The model under review builds one solid part; all positions refer to its coordinate system, in mm. Face numbers are marked on the shaded views. Give positions to 0.01 mm unless a question says otherwise; leave off trailing zeros. Loops run counter-clockwise (first coordinate to the right, second up) from the corner with the lowest first, then second, coordinate; pieces in that order, holes last. Notation, with made-up numbers: (28, 68.25) - (69, 68.25) arc R22 cw to (69, 106.25) - close; hole circle Ø2 at (-22.5, 87.5). An arc over 180 degrees is marked (long way). Return JSON: item names as keys, results as strings. Group by question number.
from build123d import *

# Parameters (mm, degrees)
SKETCH1_W           = 98
SKETCH1_H           = 60
BOSS_EXTRUDE1_DEPTH = 1.5
SKETCH2_W           = 97
SKETCH2_H           = 39.5
BOSS_EXTRUDE2_DEPTH = 9
CUT_EXTRUDE1_DEPTH  = 1.5
CUT_EXTRUDE2_REACH  = 60.155
SKETCH4_R           = 1.5
SKETCH5_W           = 37.809406893
SKETCH5_H           = 4.525576916
BOSS_EXTRUDE3_DEPTH = 0.01


with BuildPart() as part:
    # Sketch1 → Boss-Extrude1 (new body)
    with BuildSketch(Plane(origin=(0, 0, 0), x_dir=(1, 0, 0), z_dir=(0, 1, 0))):
        Rectangle(SKETCH1_W, SKETCH1_H)
    extrude(amount=BOSS_EXTRUDE1_DEPTH)

    # Sketch2 → Boss-Extrude2 (add)
    with BuildSketch(Plane(origin=(0, 1.5, 0), x_dir=(1, 0, 0), z_dir=(0, 1, 0))):
        with Locations((0, 0.25)):
            Rectangle(SKETCH2_W, SKETCH2_H)
    extrude(amount=BOSS_EXTRUDE2_DEPTH)

    # Sketch3 → Cut-Extrude1 (cut)
    with BuildSketch(Plane(origin=(0, 10.5, 0), x_dir=(1, 0, 0), z_dir=(0, 1, 0))):
        with BuildLine():
            Line((-36, 13.25), (36, 13.25))
            ThreePointArc((36, 13.25), (37.414213562, 12.664213562), (38, 11.25))
            Line((38, 11.25), (38, -10.75))
            ThreePointArc((38, -10.75), (37.414213562, -12.164213562), (36, -12.75))
            Line((36, -12.75), (-36, -12.75))
            ThreePointArc((-36, -12.75), (-37.414213562, -12.164213562), (-38, -10.75))
            Line((-38, -10.75), (-38, 11.25))
            ThreePointArc((-38, 11.25), (-37.414213562, 12.664213562), (-36, 13.25))
        make_face()
    extrude(amount=-CUT_EXTRUDE1_DEPTH, mode=Mode.SUBTRACT)

    # Sketch4 → Cut-Extrude2 (cut, up to next)
    with BuildSketch(Plane(origin=(0, 1.5, 0), x_dir=(1, 0, 0), z_dir=(0, 1, 0)), mode=Mode.PRIVATE) as cut_extrude2_sk1:
        with Locations(Location((-46.5, 27.5, 0), (0, 0, 270))):
            Circle(SKETCH4_R)
    cut_extrude2_tool1 = extrude(cut_extrude2_sk1.sketch, amount=-CUT_EXTRUDE2_REACH, mode=Mode.PRIVATE) & part.part
    # Sketch4 → Cut-Extrude2 (cut, up to next)
    with BuildSketch(Plane(origin=(0, 1.5, 0), x_dir=(1, 0, 0), z_dir=(0, 1, 0)), mode=Mode.PRIVATE) as cut_extrude2_sk2:
        with Locations(Location((46.5, 27.5, 0), (0, 0, 270))):
            Circle(SKETCH4_R)
    cut_extrude2_tool2 = extrude(cut_extrude2_sk2.sketch, amount=-CUT_EXTRUDE2_REACH, mode=Mode.PRIVATE) & part.part
    # Sketch4 → Cut-Extrude2 (cut, up to next)
    with BuildSketch(Plane(origin=(0, 1.5, 0), x_dir=(1, 0, 0), z_dir=(0, 1, 0)), mode=Mode.PRIVATE) as cut_extrude2_sk3:
        with Locations(Location((46.5, -27.5, 0), (0, 0, 270))):
            Circle(SKETCH4_R)
    cut_extrude2_tool3 = extrude(cut_extrude2_sk3.sketch, amount=-CUT_EXTRUDE2_REACH, mode=Mode.PRIVATE) & part.part
    # Sketch4 → Cut-Extrude2 (cut, up to next)
    with BuildSketch(Plane(origin=(0, 1.5, 0), x_dir=(1, 0, 0), z_dir=(0, 1, 0)), mode=Mode.PRIVATE) as cut_extrude2_sk4:
        with Locations(Location((-46.5, -27.5, 0), (0, 0, 270))):
            Circle(SKETCH4_R)
    cut_extrude2_tool4 = extrude(cut_extrude2_sk4.sketch, amount=-CUT_EXTRUDE2_REACH, mode=Mode.PRIVATE) & part.part
    add(cut_extrude2_tool1.solids().sort_by_distance((-46.5, 1.5, -27.5))[0], mode=Mode.SUBTRACT)
    add(cut_extrude2_tool2.solids().sort_by_distance((46.5, 1.5, -27.5))[0], mode=Mode.SUBTRACT)
    add(cut_extrude2_tool3.solids().sort_by_distance((46.5, 1.5, 27.5))[0], mode=Mode.SUBTRACT)
    add(cut_extrude2_tool4.solids().sort_by_distance((-46.5, 1.5, 27.5))[0], mode=Mode.SUBTRACT)

    # Sketch5 → Boss-Extrude3 (add)
    with BuildSketch(Plane(origin=(0, 1.5, 0), x_dir=(1, 0, 0), z_dir=(0, 1, 0))):
        with Locations((-21.049918021, 27.737211542)):
            Rectangle(SKETCH5_W, SKETCH5_H)
    extrude(amount=BOSS_EXTRUDE3_DEPTH)


solid = part.part
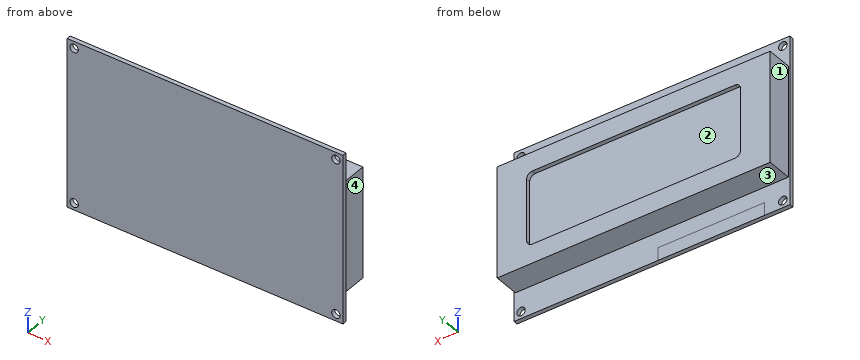
Item 1: Take a section at B-B (z = 27.5). State the section outline as (x, y) points.
Item 2: Take a section at C-C (x = 13). State the section outline as (y, z) points, then the cut area to 4 significant figures.
Item 3: Take a section at A-A (x = 46.5). State the section outline as (y, z) points, then the cut area to 4 significant figures.
Item 4: For P1, Ø3.5, axis at x = 46.5, z = 27.5, coming from the +Y side; P2, Ø4.5, axis at y = 7.5, z = 6.5, coming from the +X side; P3, Ø1, axis at x = -33.5, z = 6.5, coming from the +Y side; P4, Ø4, axis at y = 2.5, z = 6, coming from the -X side, all flat-tipped, find the tip position at first contact; note any pin that passes through.
Item 5: Take a section at D-D (z = 9). State the section outline as (x, y) points.
Item 6: Mouldability with a two-part tool opening along X and no side actions: class the marked faces 1, 2, 3 and 4 as +X half, -X half, draft (parallel to the pull), parting line (faces both ways), or undercut.
Item 7: For L1, parallel to X at y = 0.85, z = -27.5; L2, parallel to X at y = 9.5, z = 4.5; L3, parallel to Y at x = 4, z = -23.5, list the stretches that pass through material, from the lowest coordinate up. Write a range as from..to.
Check sheet entries:
{
 "1": {"outline": "(-49, 0) - (-48, 0) - (-48, 1.5) - (-49, 1.5) - close; (-45, 0) - (45, 0) - (45, 1.5) - (-45, 1.5) - close; (48, 0) - (49, 0) - (49, 1.5) - (48, 1.5) - close"},
 "2": {"outline": "(0, -30) - (1.5, -30) - (1.5, -20) - (10.5, -20) - (10.5, -13.25) - (9, -13.25) - (9, 12.75) - (10.5, 12.75) - (10.5, 19.5) - (1.5, 19.5) - (1.5, 30) - (0, 30) - close", "area": "406.5 mm^2"},
 "3": {"outline": "(0, -30) - (1.5, -30) - (1.5, -29) - (0, -29) - close; (0, -26) - (1.5, -26) - (1.5, -20) - (10.5, -20) - (10.5, 19.5) - (1.5, 19.5) - (1.5, 26) - (0, 26) - close; (0, 29) - (1.5, 29) - (1.5, 30) - (0, 30) - close", "area": "436.5 mm^2"},
 "4": {"P1": "stops at y = 1.5", "P2": "stops at x = 48.5", "P3": "stops at y = 9", "P4": "stops at x = -49"},
 "5": {"outline": "(-49, 0) - (49, 0) - (49, 1.5) - (48.5, 1.5) - (48.5, 10.5) - (38, 10.5) - (38, 9) - (-38, 9) - (-38, 10.5) - (-48.5, 10.5) - (-48.5, 1.5) - (-49, 1.5) - close"},
 "6": {"face 1": "-X half", "face 2": "undercut", "face 3": "draft", "face 4": "+X half"},
 "7": {"L1": "x = -49..-48, -45..45, 48..49", "L2": "x = -48.5..-38, 38..48.5", "L3": "y = 0..1.5"}
}
